Read the model definition and answer for the solid it produces. Units are mm, in the model's axes. A direction names the side the tool comes from. Coordinates: 2 decimals unless noted, no trailing zeros. Order: outer loops, then holes, each group sorted by start corner. A loop starts at its lowest first (then second) coordinate and runs counter-clockwise, first axis right, second up. Notation, with made-up numbers: (-32.75, -9) -> (26.25, -9) arc R7 ccw to (26.25, -2) -> close; hole circle Ø5 at (66, -21.75). An arc over 180 degrees is marked (long way). Answer as a JSON object with one key per item and string values. Group by question number.
1) Determine the mould class of faces 1 (the flat face through (9.352, 1.479, 0.084)), 2 (the flat face through (0, 1, 4)), 3 (the flat face through (0, 1, 6)) for opening direction X: released by +X, released by -X, zero draft, split by the parting line, or undercut.
2) Consider L1, parallel to Z at x = -7.5, y = 0.35; L2, parallel to X at y = 1.8, z = 0.5; L3, parallel to X at y = 2.4, z = -1.5. Determine where each line is inside the solid, lowest interval first.
3) Section B-B on x = -2.75 is taken. Determine the outline of the cut face in (y, z).
4) Section C-C on z = 2 is taken. Determine the outline of the cut face in (x, y) (3 decimals), and give its area (3 significant figures).
5) A tool of negligible diameter and unlimited length cuts with its end or side. For faces 4 (the flat face through (0, 1, -6)), 5 (the flat face through (8.36, 1.48, -0.06)), from which of +Z, -Z, +X, -X, +Y, -Y can it reach the whole face along a straight path? Write none if from no direction.
6) Section A-A on y = 2.25 is taken. Determine the outline of the cut face in (x, z), and give its area (3 significant figures).
7) Section D-D on z = -5 is taken. Determine the outline of the cut face in (x, y), and give its area (3 significant figures).
8) Given pin 1 (1.5 mm diameter, centred on y = 0.5, z = 1, fed in from +X); pin 2 (1.5 mm diameter, centred on y = 2, z = -4.5, fed in from -X), each flat-ended and moving along its own axis, determine where each tip first touches the part or whether it passes through.
from build123d import *

# Parameters (mm, degrees)
BOSS_EXTRUDE1_DEPTH = 10
BOSS_EXTRUDE2_DEPTH = 1
SKETCH3_W           = 10
SKETCH3_H           = 3
BOSS_EXTRUDE3_DEPTH = 3
FILLET1_R           = 1


with BuildPart() as part:
    # Sketch1 → Boss-Extrude1 (new body)
    with BuildSketch(Plane(origin=(0, 0, 0), x_dir=(1, 0, 0), z_dir=(0, 1, 0))):
        Polygon((-10.492426287, 6), (10.492426287, 6), (8.242426287, -6), (-8.242426287, -6), align=None)
        Polygon((-9.1, 4), (9.1, 4), (7.6, -4), (-7.6, -4), align=None, mode=Mode.SUBTRACT)
    extrude(amount=BOSS_EXTRUDE1_DEPTH)

    # Sketch2 → Boss-Extrude2 (add)
    with BuildSketch(Plane(origin=(0, 10, 0), x_dir=(1, 0, 0), z_dir=(0, 1, 0))):
        Polygon((-10.492426287, 6), (-8.242426287, -6), (8.242426287, -6), (10.492426287, 6), align=None)
    extrude(amount=BOSS_EXTRUDE2_DEPTH)

    # Sketch3 → Boss-Extrude3 (add)
    with BuildSketch(Plane(origin=(0, 11, 0), x_dir=(1, 0, 0), z_dir=(0, 1, 0))):
        with Locations((0, 7.5)):
            Rectangle(SKETCH3_W, SKETCH3_H)
        with Locations((0, -7.5)):
            Rectangle(SKETCH3_W, SKETCH3_H)
    extrude(amount=-BOSS_EXTRUDE3_DEPTH)

    # Fillet1
    fillet1_edges = [part.edges().sort_by_distance(p)[0] for p in [
        (-5, 9.5, 9),
        (-5, 8, 7.5),
        (5, 8, 7.5),
        (5, 9.5, 9),
        (5, 9.5, -9),
        (5, 8, -7.5),
        (-5, 8, -7.5),
        (-5, 9.5, -9),
        (0, 8, -9),
        (0, 8, 9),
        (-5, 9.5, 6),
        (5, 9.5, 6),
        (0, 8, 6),
        (5, 9.5, -6),
        (-5, 9.5, -6),
        (0, 8, -6),
    ]]
    fillet(fillet1_edges, radius=FILLET1_R)

    # Split1
    split(bisect_by=Plane(origin=(0, 3, 0), x_dir=(0, 0, -1), z_dir=(0, -1, 0)), keep=Keep.TOP)


solid = part.part
Worked answers:
{
 "1": {"face 1": "released by +X", "face 2": "undercut", "face 3": "zero draft"},
 "2": {"L1": "z = -6 to -4, 4 to 6", "L2": "x = -9.27 to -8.26, 8.26 to 9.27", "L3": "x = -9.65 to -8.63, 8.63 to 9.65"},
 "3": {"outline": "(0, -6) -> (3, -6) -> (3, -4) -> (0, -4) -> close; (0, 4) -> (3, 4) -> (3, 6) -> (0, 6) -> close"},
 "4": {"outline": "(-8.992, 0) -> (-7.975, 0) -> (-7.975, 3) -> (-8.992, 3) -> close; (7.975, 0) -> (8.992, 0) -> (8.992, 3) -> (7.975, 3) -> close", "area": "6.10 mm²"},
 "5": {"face 4": "-Z, +X, -X, +Y, -Y", "face 5": "+Y, -Y"},
 "6": {"outline": "(-10.49, -6) -> (10.49, -6) -> (8.24, 6) -> (-8.24, 6) -> close; hole (-9.1, -4) -> (9.1, -4) -> (7.6, 4) -> (-7.6, 4) -> close", "area": "91.2 mm²"},
 "7": {"outline": "(-10.3, 0) -> (10.3, 0) -> (10.3, 3) -> (-10.3, 3) -> close", "area": "61.8 mm²"},
 "8": {"pin 1": "stops at x = 9.32", "pin 2": "stops at x = -10.35"}
}
